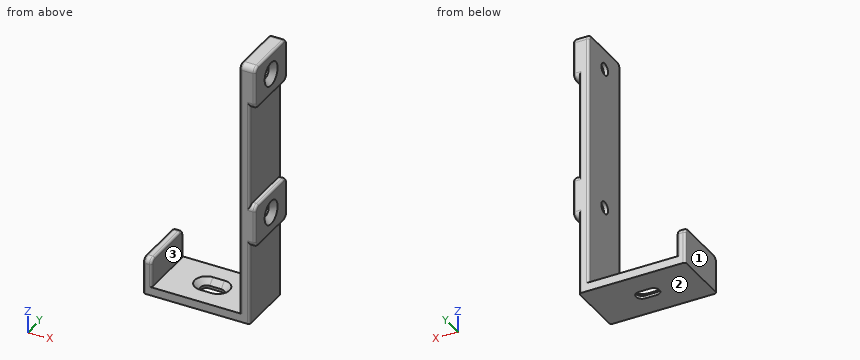
from build123d import *

# Parameters (mm, degrees)
SKETCH013_W         = 30.5
SKETCH013_H         = 20
PAD007_DEPTH        = 3
PAD008_DEPTH        = 3
PAD009_DEPTH        = 3.5
HOLE004_D           = 4.2
HOLE004_DEPTH       = 25
HOLE004_CSINK_D     = 8.4
HOLE004_CSINK_ANGLE = 90
HOLE004_TIPS_R      = 2.1
POCKET002_DEPTH     = 3.001
CHAMFER_SIZE        = 2
FILLET_R            = 0.8
PAD017_DEPTH        = 2
HOLE008_D           = 4.2
HOLE008_DEPTH       = 25
HOLE008_CSINK_D     = 8.2
HOLE008_CSINK_ANGLE = 90
HOLE008_TIPS_R      = 2.1
FILLET002_R         = 0.8


with BuildPart() as part:
    # Sketch013 → Pad007 (new body)
    with BuildSketch(Plane.XY):
        with Locations((18.25, 10)):
            Rectangle(SKETCH013_W, SKETCH013_H)
    extrude(amount=PAD007_DEPTH)

    # Sketch014 (on Face4 of Pad007) → Pad008 (join)
    with BuildSketch(Plane(origin=(3, 0, 0), x_dir=(0, -1, 0), z_dir=(-1, 0, 0))):
        with BuildLine():
            Line((-20, 0), (0, 0))
            Line((0, 0), (0, 11))
            ThreePointArc((0, 11), (-0.585786, 12.414214), (-2, 13))
            Line((-2, 13), (-18, 13))
            ThreePointArc((-18, 13), (-19.414214, 12.414214), (-20, 11))
            Line((-20, 11), (-20, 0))
        make_face()
    extrude(amount=PAD008_DEPTH)

    # Sketch015 (on Face1 of Pad008) → Pad009 (join)
    with BuildSketch(Plane.YZ.offset(33.5)):
        with BuildLine():
            Line((20, 0), (20, 91))
            ThreePointArc((20, 91), (19.414214, 92.414214), (18, 93))
            Line((18, 93), (2, 93))
            ThreePointArc((2, 93), (0.585786, 92.414214), (0, 91))
            Line((0, 91), (0, 0))
            Line((0, 0), (20, 0))
        make_face()
    extrude(amount=PAD009_DEPTH)

    # Hole004
    with Locations(Plane.YZ.offset(37)):
        with Locations((10, 35.5), (10, 85.5)):
            CounterSinkHole(HOLE004_D / 2, HOLE004_CSINK_D / 2, depth=HOLE004_DEPTH, counter_sink_angle=HOLE004_CSINK_ANGLE)

    # Hole004 tips → Hole004 tip 1 section 0
    with BuildSketch(Plane.YZ.offset(12), mode=Mode.PRIVATE) as hole004_tip_1_s0:
        with Locations((10, 35.5)):
            Circle(HOLE004_TIPS_R)
    loft([hole004_tip_1_s0.sketch, Vertex(10.738193, 10, 35.5)], mode=Mode.SUBTRACT)

    # Hole004 tips → Hole004 tip 2 section 0
    with BuildSketch(Plane.YZ.offset(12), mode=Mode.PRIVATE) as hole004_tip_2_s0:
        with Locations((10, 85.5)):
            Circle(HOLE004_TIPS_R)
    loft([hole004_tip_2_s0.sketch, Vertex(10.738193, 10, 85.5)], mode=Mode.SUBTRACT)

    # Sketch017 (on Face1 of Hole004) → Pocket002 (cut, through all)
    with BuildSketch(Plane.XY.offset(3)):
        with BuildLine():
            ThreePointArc((16.553834, 12.053193), (14.478422, 9.977781), (16.553834, 7.902369))
            Line((16.553834, 7.902369), (20.553834, 7.902369))
            ThreePointArc((20.553834, 7.902369), (22.629246, 9.977781), (20.553834, 12.053193))
            Line((16.553834, 12.053193), (20.553834, 12.053193))
        make_face()
    extrude(amount=-POCKET002_DEPTH, mode=Mode.SUBTRACT)

    # Chamfer
    chamfer_edges = [part.edges().sort_by_distance(p)[0] for p in [
        (18.553834, 7.902369, 3),
    ]]
    chamfer(chamfer_edges, length=CHAMFER_SIZE)

    # Fillet
    fillet_edges = [part.edges().sort_by_distance(p)[0] for p in [
        (0, 10, 13),
        (3, 10, 13),
        (33.5, 10, 93),
        (37, 10, 93),
    ]]
    fillet(fillet_edges, radius=FILLET_R)

    # Sketch035 (on Face38 of Fillet) → Pad017 (join, symmetric)
    with BuildSketch(Plane.YZ.offset(37)):
        with BuildLine():
            Line((0, 91), (0, 80))
            ThreePointArc((0, 80), (0.585786, 78.585786), (2, 78))
            Line((2, 78), (18, 78))
            ThreePointArc((18, 78), (19.414214, 78.585786), (20, 80))
            Line((20, 80), (20, 91))
            ThreePointArc((20, 91), (19.414214, 92.414214), (18, 93))
            Line((18, 93), (2, 93))
            ThreePointArc((2, 93), (0.585786, 92.414214), (0, 91))
        make_face()
        with BuildLine():
            Line((0, 41), (0, 30))
            ThreePointArc((0, 30), (0.585786, 28.585786), (2, 28))
            Line((2, 28), (18, 28))
            ThreePointArc((18, 28), (19.414214, 28.585786), (20, 30))
            Line((20, 30), (20, 41))
            ThreePointArc((20, 41), (19.414214, 42.414214), (18, 43))
            Line((18, 43), (2, 43))
            ThreePointArc((2, 43), (0.585786, 42.414214), (0, 41))
        make_face()
    extrude(amount=PAD017_DEPTH, both=True)

    # Hole008
    with Locations(Plane.YZ.offset(39)):
        with Locations((10, 85.5), (10, 35.5)):
            CounterSinkHole(HOLE008_D / 2, HOLE008_CSINK_D / 2, depth=HOLE008_DEPTH, counter_sink_angle=HOLE008_CSINK_ANGLE)

    # Hole008 tips → Hole008 tip 1 section 0
    with BuildSketch(Plane.YZ.offset(14), mode=Mode.PRIVATE) as hole008_tip_1_s0:
        with Locations((10, 85.5)):
            Circle(HOLE008_TIPS_R)
    loft([hole008_tip_1_s0.sketch, Vertex(12.738193, 10, 85.5)], mode=Mode.SUBTRACT)

    # Hole008 tips → Hole008 tip 2 section 0
    with BuildSketch(Plane.YZ.offset(14), mode=Mode.PRIVATE) as hole008_tip_2_s0:
        with Locations((10, 35.5)):
            Circle(HOLE008_TIPS_R)
    loft([hole008_tip_2_s0.sketch, Vertex(12.738193, 10, 35.5)], mode=Mode.SUBTRACT)

    # Fillet002
    fillet002_edges = [part.edges().sort_by_distance(p)[0] for p in [
        (39, 10, 93),
        (39, 10, 43),
    ]]
    fillet(fillet002_edges, radius=FILLET002_R)


with BuildPart() as part_1:
    # Body003 placement: moved
    add(part.part.moved(Location((-104.9, 0, 0))))


solid = part_1.part
The listing builds one solid part. Answer for the finished solid, in the listing's coordinates (mm). Face numbers are marked on the shaded views. Coordinates: 2 decimals unless noted, no trailing zeros. Loops run counter-clockwise (first coordinate to the right, second up) from the corner with the lowest first, then second, coordinate; pieces in that order, holes last. Notation, with made-up numbers: (-32.5, 45.5) -> (-15.5, 45.5) arc R21 cw to (-15.5, 52.5) -> close; hole circle Ø7 at (68, -18.75). An arc over 180 degrees is marked (long way). Write item = value, one per line. Start each with the question number.
1) A cutting plane is placed at D-D (z = 15). Give the vertices of the cut face in (x, y), then the cut area to 3 significant figures.
2) Given pin 1 Ø4.5 at (y, z) = (10, 8.5) entering from +X; pin 2 Ø0.6 at (x, y) = (-67, 13) entering from -Z; pin 3 Ø3.5 at (y, z) = (9, 36) entering from -X, each flat-ended and moving along its own axis, determine where each tip first touches the part or whether it passes through.
3) A cutting plane is placed at B-B (x = -85.5). Give the vertices of the cut face in (y, z).
4) A cutting plane is placed at A-A (z = 85.5). Give the vertices of the cut face in (x, y).
5) Straight lines are drawn through the part: line 1 (Z direction, x = -68.5, y = 10.25); line 2 (Y direction, x = -70.45, z = 35.5); line 3 (X direction, y = 18, z = 13.5). For each, find the intervals that lie inside material, in ascending order. Write a range as from..to.
6) The mould has two halves that part along X. Classify the marked faces 1, 2 and 3: released by +X, released by -X, zero draft, split by the parting line, or undercut.
7) A cutting plane is placed at C-C (y = 4.25). Give the vertices of the cut face in (x, z).
Responses:
q1.outline = (-71.4, 0.8) arc R0.8 ccw to (-70.6, 0) -> (-68.7, 0) arc R0.8 ccw to (-67.9, 0.8) -> (-67.9, 19.2) arc R0.8 ccw to (-68.7, 20) -> (-70.6, 20) arc R0.8 ccw to (-71.4, 19.2) -> close
q1.area = 69.5 mm²
q2.pin_1 = -67.9
q2.pin_2 = 28
q2.pin_3 = -71.4
q3.outline = (0, 0) -> (7.9, 0) -> (7.9, 1) -> (5.9, 3) -> (0, 3) -> close; (12.05, 0) -> (20, 0) -> (20, 3) -> (14.05, 3) -> (12.05, 1) -> close
q4.outline = (-71.4, 0.8) arc R0.8 ccw to (-70.6, 0) -> (-66.7, 0) arc R0.8 ccw to (-65.9, 0.8) -> (-65.9, 5.9) -> (-67.9, 7.9) -> (-69.9, 7.9) -> (-69.9, 7.8) -> (-70, 7.9) -> (-71.4, 7.9) -> close; (-71.4, 12.1) -> (-70, 12.1) -> (-69.9, 12.2) -> (-69.9, 12.1) -> (-67.9, 12.1) -> (-65.9, 14.1) -> (-65.9, 19.2) arc R0.8 ccw to (-66.7, 20) -> (-70.6, 20) arc R0.8 ccw to (-71.4, 19.2) -> close
q5.line_1 = 0..33.41, 37.59..83.41, 87.59..93
q5.line_2 = 0..7.9, 12.1..20
q5.line_3 = -71.4..-67.9
q6.face_1 = released by -X
q6.face_2 = zero draft
q6.face_3 = undercut
q7.outline = (-104.9, 0) -> (-67.9, 0) -> (-67.9, 28) -> (-66.7, 28) arc R0.8 ccw to (-65.9, 28.8) -> (-65.9, 42.2) arc R0.8 ccw to (-66.7, 43) -> (-67.9, 43) -> (-67.9, 78) -> (-66.7, 78) arc R0.8 ccw to (-65.9, 78.8) -> (-65.9, 92.2) arc R0.8 ccw to (-66.7, 93) -> (-70.6, 93) arc R0.8 ccw to (-71.4, 92.2) -> (-71.4, 3) -> (-101.9, 3) -> (-101.9, 12.2) arc R0.8 ccw to (-102.7, 13) -> (-104.1, 13) arc R0.8 ccw to (-104.9, 12.2) -> close
